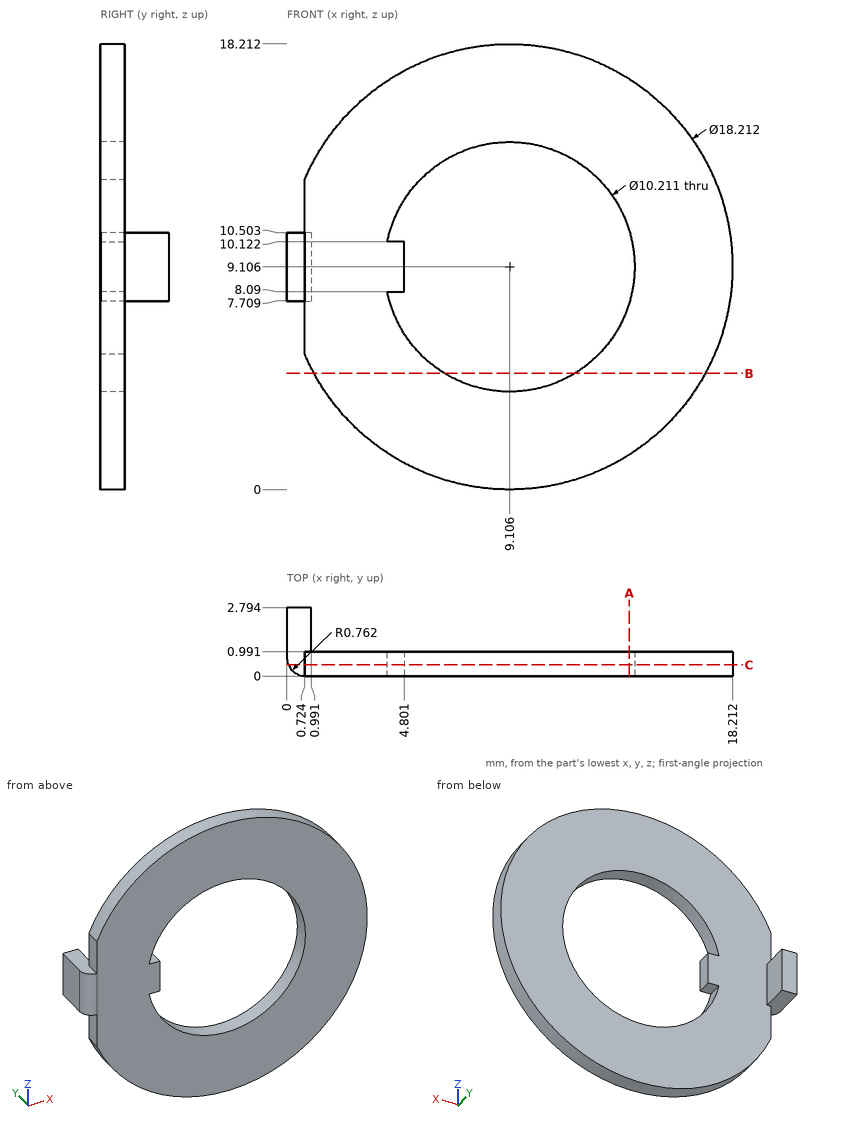
Part print with two shaded views. Sizes in mm from the minimum x, y, z corner. Round coordinates to 2 decimals unless told otherwise and drop trailing zeros. Order: outer loops, then holes, each group sorted by start corner. A loop starts at its lowest first (then second) coordinate and runs counter-clockwise, first axis right, second up. Notation, with made-up numbers: (-34, -29.75) - (19, -29.75) arc R19 cw to (19, -19.75) - close; hole circle Ø5 at (70.5, 9.25). An arc over 180 degrees is marked (long way). Answer as CSV lines item,"result". Start each with the question number.
1. Pin check, flat tips, straight feed: pin 1 (8.5 mm diameter, centred on x = 5.5, z = 5, fed in from +Y); pin 2 (1.5 mm diameter, centred on x = 6.5, z = 2, fed in from -Y); pin 3 (4 mm diameter, centred on x = 11, z = 7, fed in from +Y); pin 4 (1.4 mm diameter, centred on y = 2.5, z = 9, fed in from +X). Stop position of each tip, or through.
2. Saw through at B-B, the plane z = 4.75. Write the cut outline in (x, y).
3. Saw through at C-C, the plane y = 0.45. Write the cut outline in (x, z) (1 decimal).
4. Saw through at A-A, the plane x = 14. Write the cut outline in (y, z) (1 decimal).
5. Drill centre lines: L1, parallel to X at y = 0.65, z = 8 (1 decimal); L2, parallel to Y at x = 10.25, z = 2.5; L3, parallel to Z at x = 7, y = 0.35 (1 decimal). Where is each one in solid material? Low to high. Write a range as [from, to].
Model answer:
1,pin 1,"stops at y = 0.99"
1,pin 2,"stops at y = 0"
1,pin 3,"passes through"
1,pin 4,"stops at x = 0.99"
2,outline,"(1.11, 0) - (6.44, 0) - (6.44, 0.99) - (1.11, 0.99) - close; (11.77, 0) - (17.1, 0) - (17.1, 0.99) - (11.77, 0.99) - close"
3,outline,"(0.1, 7.7) - (0.7, 7.7) - (0.7, 5.5) arc R9.1 ccw (long way) to (0.7, 12.7) - (0.7, 10.5) - (0.1, 10.5) - close; hole (4.1, 8.1) arc R5.1 ccw (long way) to (4.1, 10.1) - (4.8, 10.1) - (4.8, 8.1) - close"
4,outline,"(0, 1.4) - (1, 1.4) - (1, 7.7) - (0, 7.7) - close; (0, 10.6) - (1, 10.6) - (1, 16.8) - (0, 16.8) - close"
5,L1,"x = [0, 4.1], [14.1, 18.1]"
5,L2,"y = [0, 0.99]"
5,L3,"z = [0.2, 4.5], [13.8, 18]"
